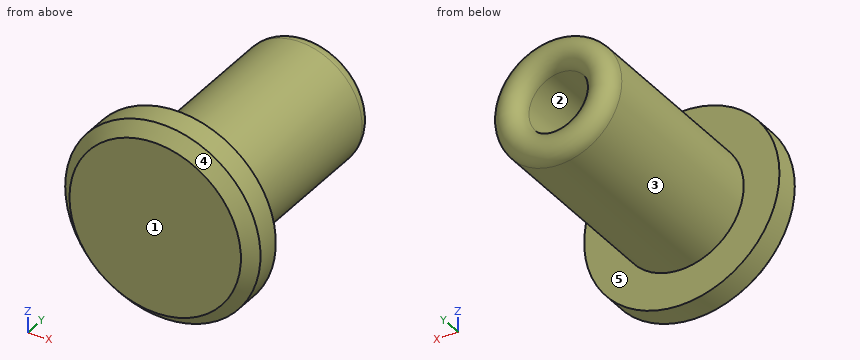
```python
from build123d import *

# Parameters (mm, degrees)
CHAMFER1_SIZE = 0.5


with BuildPart() as part:
    # Sketch1 → Revolve1 (revolve)
    with BuildSketch(Plane.XY):
        with BuildLine():
            Line((0, 0), (0, 0.5))
            Line((0, 0.5), (-0.3, 0.5))
            ThreePointArc((-0.3, 0.5), (-1.007106781, 0.792893219), (-1.3, 1.5))
            Line((-1.3, 1.5), (-1.3, 9.45))
            ThreePointArc((-1.3, 9.45), (-1.95, 10.1), (-2.6, 9.45))
            Line((-2.6, 9.45), (-2.6, 1.5))
            Line((-2.6, 1.5), (-4.1, 1.5))
            Line((-4.1, 1.5), (-4.1, 0))
            Line((-4.1, 0), (0, 0))
        make_face()
    revolve(axis=Axis((0, -1000, 0), (0, 1, 0)))

    # Chamfer1
    chamfer1_edges = [part.edges().sort_by_distance(p)[0] for p in [
        (4.1, 0, 0),
    ]]
    chamfer(chamfer1_edges, length=CHAMFER1_SIZE)


solid = part.part
```
Here's how the part is built. I have some questions about the finished solid (model axes, mm). Face numbers are marked on the shaded views. A direction names the side the tool comes from. Coordinates: 2 decimals unless noted, no trailing zeros. Order: outer loops, then holes, each group sorted by start corner. A loop starts at its lowest first (then second) coordinate and runs counter-clockwise, first axis right, second up.
1) I need wall thicknesses on line 1 (Z direction, x = 0, y = 4.5); line 2 (Z direction, x = -2.25, y = 8.25); line 3 (Y direction, x = 3, z = -0.75). Which ranges of each line are inside material? Lowest first, please.
2) Will these pins go through, and if not, where does the flat tip stop? pin 1 (2 mm diameter, centred on x = 0, y = 4, fed in from -Z); pin 2 (2 mm diameter, centred on y = 2, z = -3, fed in from -X); pin 3 (2 mm diameter, centred on x = 0, z = 0, fed in from +Y).
3) We'd pull the mould along X, two halves only. Please class the marked faces 1, 2 and 3: +X half, -X half, draft (parallel to the pull), parting line (faces both ways), or undercut.
4) Which directions (+Z, -Z, +X, -X, +Y, -Y) give clear straight access to the entire face, cutting with the end or side of a thin tool? Please do the marked faces 4 and 5.
5) Imagine slicing it at A-A on y = 5.5. List the corners of the cut face in (x, z) for me, and give its area (3 significant figures).
Response values:
1. line 1: z = -2.6 to -1.3, 1.3 to 2.6
1. line 2: z = -1.3 to 1.3
1. line 3: y = 0 to 1.5
2. pin 1: stops at z = -2.6
2. pin 2: stops at x = -3.5
2. pin 3: stops at y = 0.79
3. face 1: draft
3. face 2: undercut
3. face 3: parting line
4. face 4: -Y
4. face 5: +Y
5. outline: circle Ø5.2 at (0, 0); hole circle Ø2.6 at (0, 0)
5. area: 15.9 mm2
